The drawing under review shows one solid part. Ordinate dimensions are in mm from its lowest x, y, z. A direction names the side the tool comes from. Give positions to 0.01 mm unless a question says otherwise; leave off trailing zeros. Order: outer loops, then holes, each group sorted by start corner. A loop starts at its lowest first (then second) coordinate and runs counter-clockwise, first axis right, second up. Notation, with made-up numbers: (-9, 45) - (1, 45) arc R23 ccw to (1, 59) - close; hole circle Ø11 at (89.25, 42). An arc over 180 degrees is marked (long way). Use CSV: the item, a comma, the result in double quotes.
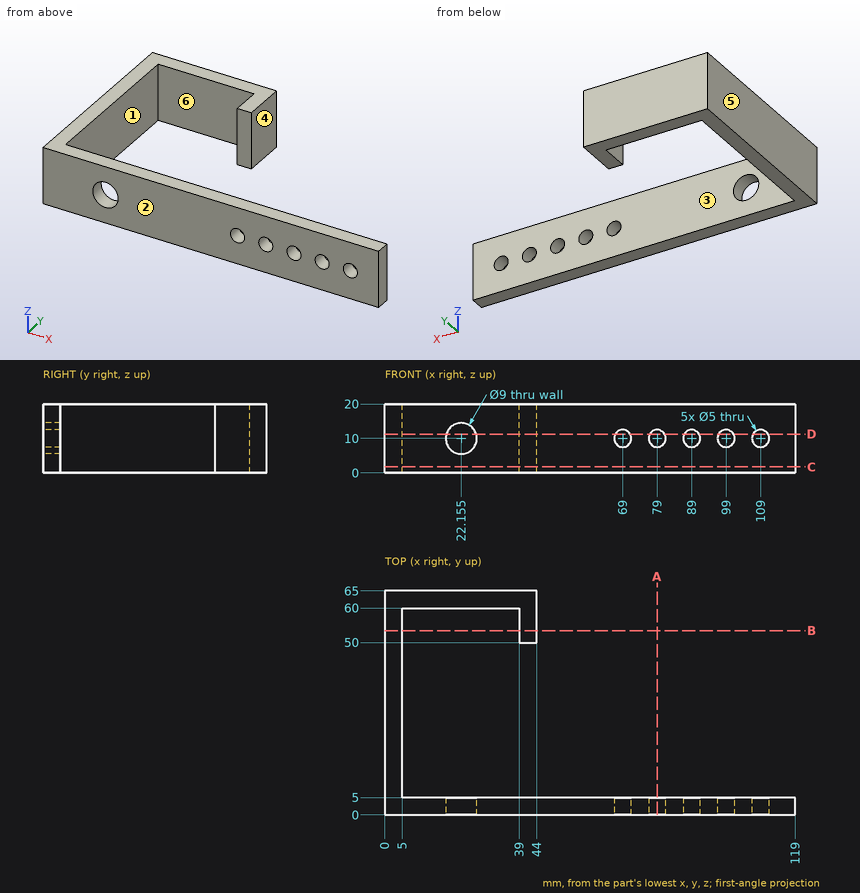
Item 1: Mouldability with a two-part tool opening along X and no side actions: class the marked faces 3, 4, 5 and 6 as pulls with the +X half, pulls with the -X half, needs draft (parallel to the pull), parting line crosses it, or undercut.
Results list:
face 3,"needs draft"
face 4,"pulls with the +X half"
face 5,"pulls with the -X half"
face 6,"undercut"
Item 2: Wall thickness on L1, parallel to Y at x = 28.5, z = 16.5; L2, parallel to X at y = 55, z = 12; L3, parallel to Z at x = 89, y = 2.2: over which ranges is each line inside the solid? List them lowest first.
Results list:
L1,"y = 0 to 5, 60 to 65"
L2,"x = 0 to 5, 39 to 44"
L3,"z = 0 to 7.5, 12.5 to 20"
Item 3: Take a section at C-C, the plane z = 1.75. Give the boundary of the cut face in (x, y).
Results list:
outline,"(0, 0) - (119, 0) - (119, 5) - (5, 5) - (5, 60) - (39, 60) - (39, 50) - (44, 50) - (44, 65) - (0, 65) - close"
Item 4: Tool access review of the marked faces 1 and 2: name each direction out of +Z, -Z, +X, -X, +Y, -Y from which nothing blocks a thin tool from reaching the whole face with its end or side.
Results list:
face 1,"+Z, -Z"
face 2,"+Z, -Z, +X, -X, -Y"
Item 5: Take a section at B-B, the plane y = 53.5. Give the boundary of the cut face in (x, z).
Results list:
outline,"(0, 0) - (5, 0) - (5, 20) - (0, 20) - close; (39, 0) - (44, 0) - (44, 20) - (39, 20) - close"
Item 6: Take a section at D-D, the plane z = 11.25. State how many separate pieces and enclosed holes the cut face has.
Results list:
separate pieces,"7"
enclosed holes,"0"
Item 7: Clearance check with flat-ended pins moving along their axes: pin 1 (7 mm diameter, centred on x = 22.15, z = 10, fed in from -Y); pin 2 (6 mm diameter, centred on y = 40.5, z = 9, fed in from +X); pin 3 (3 mm diameter, centred on x = 89, z = 10, fed in from -Y); pin 4 (12 mm diameter, centred on y = 57.5, z = 5.5, fed in from +X). State where each tip first meets the part, or that it passes through.
Results list:
pin 1,"stops at y = 60"
pin 2,"stops at x = 5"
pin 3,"passes through"
pin 4,"stops at x = 44"
Item 8: Take a section at A-A, the plane x = 79. Give the boundary of the cut face in (y, z), and give its area (3 significant figures).
Results list:
outline,"(0, 0) - (5, 0) - (5, 7.5) - (0, 7.5) - close; (0, 12.5) - (5, 12.5) - (5, 20) - (0, 20) - close"
area,"75.0 mm2"
